Design review of the part shown in the three views and the two pictorial views. Dimensions are in mm from the part's minimum x, y and z. A direction names the side the tool comes from. Coordinates: 2 decimals unless noted, no trailing zeros. Loops run counter-clockwise (first coordinate to the right, second up) from the corner with the lowest first, then second, coordinate; pieces in that order, holes last. Notation, with made-up numbers: (32.25, -8) -> (72.25, -8) arc R12 ccw to (72.25, 4) -> close; hole circle Ø4 at (-20, 83). An arc over 180 degrees is marked (long way). Answer in a Markdown table with one row per item.
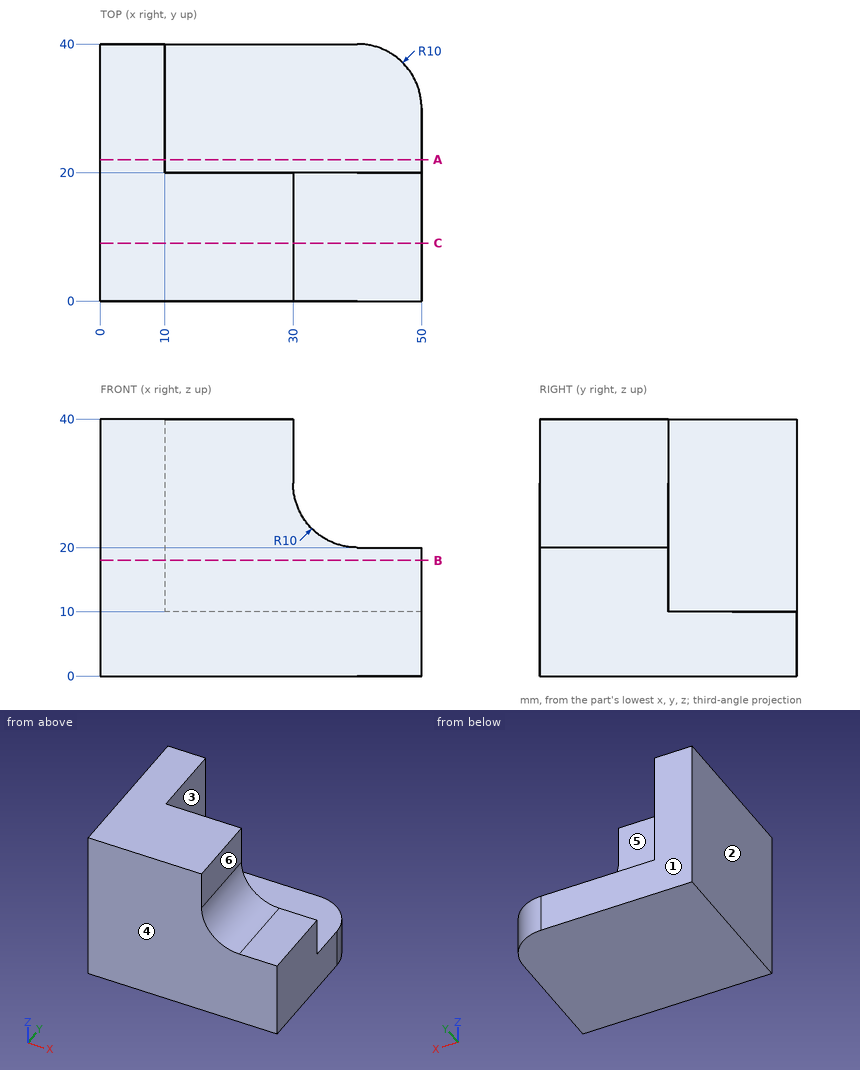
Item 1: Take a section at C-C, the plane y = 9. State the section outline as (x, z) points.
Worked answers:
| item | result |
|---|---|
| outline | (0, 0) -> (50, 0) -> (50, 20) -> (40, 20) arc R10 cw to (30, 30) -> (30, 40) -> (0, 40) -> close |
Item 2: Take a section at B-B, the plane z = 18. State the section outline as (x, y) points.
Worked answers:
| item | result |
|---|---|
| outline | (0, 0) -> (50, 0) -> (50, 20) -> (10, 20) -> (10, 40) -> (0, 40) -> close |
Item 3: The part is to be moulded in two halves that separate along X. For the marked faces 1, 2 and 3, say which applies: +X half, -X half, draft (parallel to the pull), parting line (faces both ways), or undercut.
Worked answers:
| item | result |
|---|---|
| face 1 | draft |
| face 2 | -X half |
| face 3 | +X half |
Item 4: For the marked faces 4, 5 and 6, list the 3-axis set-ups (+Z, -Z, +X, -X, +Y, -Y) from which the entire face can be reached by the end or side of a thin tool; tool diameter is ignored.
Worked answers:
| item | result |
|---|---|
| face 4 | +Z, -Z, +X, -X, -Y |
| face 5 | +Z, +X, +Y |
| face 6 | +Z, +X, +Y, -Y |
Item 5: For L1, parallel to X at y = 4, z = 34.5; L2, parallel to Y at x = 30, z = 24; L3, parallel to Z at x = 47, y = 35, list the stretches that pass through material, from the lowest coordinate up.
Worked answers:
| item | result |
|---|---|
| L1 | 0 to 30 |
| L2 | 0 to 20 |
| L3 | 0 to 10 |
Item 6: Insertion check: pin 1 (8 mm diameter, centred on y = 7, z = 34.5, fed in from +X); pin 2 (10 mm diameter, centred on x = 32, y = 35, fed in from +Z); pin 3 (12 mm diameter, centred on x = 35.5, z = 20, fed in from +Y). Each pin has a flat end and moves straight along its axis. Give the tip position at first contact, or say it passes through.
Worked answers:
| item | result |
|---|---|
| pin 1 | x = 30 |
| pin 2 | z = 10 |
| pin 3 | y = 20 |
Item 7: Take a section at A-A, the plane y = 22. State the section outline as (x, z) points.
Worked answers:
| item | result |
|---|---|
| outline | (0, 0) -> (50, 0) -> (50, 10) -> (10, 10) -> (10, 40) -> (0, 40) -> close |
